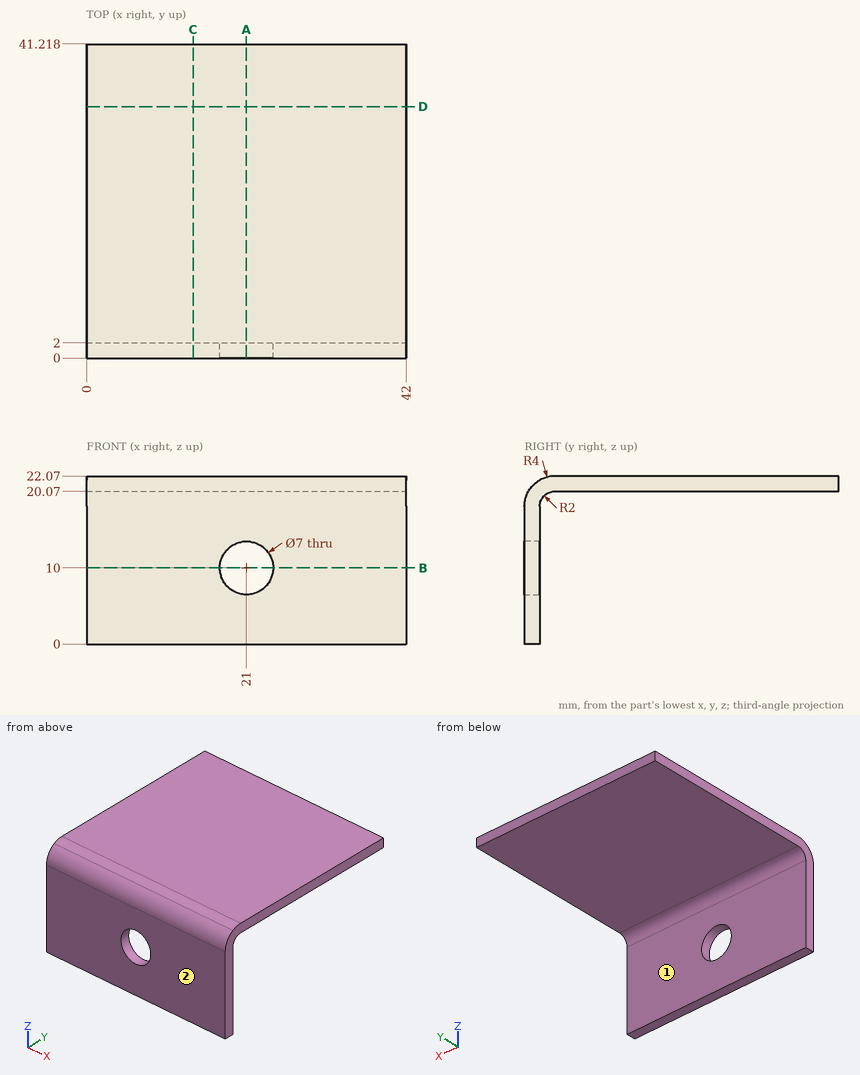
Job drawing, mm, ordinate dimensions from the low corner. One solid piece. A direction names the side the tool comes from. Round coordinates to 2 decimals unless told otherwise and drop trailing zeros. Write each loop counter-clockwise with the first axis right and the second up, starting at its lowest first coordinate (ties: lowest second). Pieces come first, ordered by that corner, then holes. Notation, with made-up numbers: M -32.75,77.5 L -19.75,77.5 A22 cw -19.75,85.5 Z; hole C 64,22.5 d7. An arc over 180 degrees is marked long. Return JSON: item names as keys, results as strings. Group by question number.
(1) Drill centre lines: probe 1 along X at (y, z) = (1.25, 10); probe 2 along Z at (x, y) = (12, 20); probe 3 along Y at (x, z) = (17, 14). Where is each one in solid material? Low to high.
(2) Saw through at C-C on x = 14. Write the cut outline in (y, z).
(3) Saw through at A-A on x = 21. Write the cut outline in (y, z).
(4) Pin check, flat tips, straight feed: pin 1 Ø9 at (x, z) = (21, 10) entering from -Y; pin 2 Ø1.5 at (x, y) = (35, 7) entering from -Z; pin 3 Ø1.5 at (x, z) = (8, 12) entering from +Y. Stop position of each tip, or through.
(5) Which spindle directions (+Z, -Z, +X, -X, +Y, -Y) get a long thin tool onto all of the face, cutting with end or side? Do the marked faces 1 and 2. Say none if no direction does.
(6) Saw through at D-D on y = 33. Write the cut outline in (x, z).
(7) Saw through at B-B on z = 10. Write the cut outline in (x, y).
Returned:
{
 "1": {"probe 1": "0 to 17.5, 24.5 to 42", "probe 2": "20.07 to 22.07", "probe 3": "0 to 2"},
 "2": {"outline": "M 0,0 L 2,0 L 2,18.07 A2 cw 4,20.07 L 41.22,20.07 L 41.22,22.07 L 4,22.07 A4 ccw 0,18.07 Z"},
 "3": {"outline": "M 0,0 L 2,0 L 2,6.5 L 0,6.5 Z; M 0,13.5 L 2,13.5 L 2,18.07 A2 cw 4,20.07 L 41.22,20.07 L 41.22,22.07 L 4,22.07 A4 ccw 0,18.07 Z"},
 "4": {"pin 1": "y = 0", "pin 2": "z = 20.07", "pin 3": "y = 2"},
 "5": {"face 1": "-Z, +X, -X, +Y", "face 2": "+Z, -Z, +X, -X, -Y"},
 "6": {"outline": "M 0,20.07 L 42,20.07 L 42,22.07 L 0,22.07 Z"},
 "7": {"outline": "M 0,0 L 17.5,0 L 17.5,2 L 0,2 Z; M 24.5,0 L 42,0 L 42,2 L 24.5,2 Z"}
}
